Here's how the part is built. I have some questions about the finished solid (model axes, mm). A direction names the side the tool comes from. Give positions to 0.01 mm unless a question says otherwise; leave off trailing zeros. Loops run counter-clockwise (first coordinate to the right, second up) from the corner with the lowest first, then second, coordinate; pieces in that order, holes last. Notation, with made-up numbers: (61.5, -16) - (82.5, -16) arc R17 ccw to (82.5, 16) - close; hole circle Ø11 at (-20, 58). An arc over 180 degrees is marked (long way). Return JSON: item names as keys, results as strings. Group by question number.
(1) I need wall thicknesses on probe 1 along X at (y, z) = (12.75, -0.1); probe 2 along Y at (x, z) = (-1.5, 0.95); probe 3 along Z at (x, y) = (-0.5, 22). Which ranges of each line are inside material? Lowest first, please. Write a range as [from, to].
(2) If we section it at C-C (z = 1.25): Please give me the cut outline in (x, y), then the cut area to 3 significant figures.
(3) If we mould it in two halves opening along Y, with no side actions, what happens to faces 1 (the cylindrical face through (1, 10, 0)), 2 (the flat face through (1, 22.209, 1)), 3 (the flat face through (1, 20, 1))? For each: released by +Y, released by -Y, zero draft, split by the parting line, or undercut.
(4) On a 3-axis mill with a long thin cutter (end or side, diameter ignored), from which of +Z, -Z, +X, -X, +Y, -Y can I reach the whole of each face in a straight line? I mean faces 4 (the cylindrical face through (1, 22, 0)), 5 (the cylindrical face through (2, 21, 0)). Say none if no direction works.
(5) For P1, Ø2, axis at y = 4.5, z = -1.5, coming from the +X side; P2, Ø2, axis at y = 17.5, z = 0, coming from the +X side, each with a flat end and sliding along its axis, tell me the tip position at first contact or that it passes through.
(6) If we section it at A-A (x = 0): Please give me the cut outline in (y, z), then the cut area to 3 significant figures.
(7) If we section it at D-D (y = 9.75): Please give me the cut outline in (x, z).
(8) If we section it at B-B (z = 0): Please give me the cut outline in (x, y), then the cut area to 3 significant figures.
```python
from build123d import *


with BuildPart() as part:
    # Sketch1 → Screw Revolve (revolve)
    with BuildSketch(Plane.XY, mode=Mode.PRIVATE) as screw_revolve_sk:
        with BuildLine():
            Line((0, 0), (1, 0))
            Line((1, 0), (1, 20))
            Line((1, 20), (2, 20))
            Line((2, 20), (2, 21.209302326))
            Line((2, 21.209302326), (1, 21.209302326))
            Line((1, 21.209302326), (1, 22.209302326))
            Line((1, 22.209302326), (2, 22.209302326))
            ThreePointArc((2, 22.209302326), (1.414213562, 23.623515888), (0, 24.209302326))
            Line((0, 24.209302326), (0, 0))
        make_face()
    revolve(screw_revolve_sk.sketch.rotate(Axis((0, 0, 0), (0, 1, 0)), 90), axis=Axis((0, 0, 0), (0, 1, 0)))


solid = part.part
```
Values:
{
 "1": {"probe 1": "[-0.99, 0.99]", "probe 2": "[20, 21.21], [22.21, 23.13]", "probe 3": "[-0.87, 0.87]"},
 "2": {"outline": "(-1.56, 20) - (1.56, 20) - (1.56, 21.21) - (-1.56, 21.21) - close; (-1.56, 22.21) - (1.56, 22.21) arc R1.56 ccw to start", "area": "7.60 mm2"},
 "3": {"face 1": "zero draft", "face 2": "undercut", "face 3": "released by -Y"},
 "4": {"face 4": "none", "face 5": "+Y, -Y"},
 "5": {"P1": "x = 0.87", "P2": "x = 1"},
 "6": {"outline": "(0, -1) - (20, -1) - (20, -2) - (21.21, -2) - (21.21, -1) - (22.21, -1) - (22.21, -2) arc R2 ccw to (22.21, 2) - (22.21, 1) - (21.21, 1) - (21.21, 2) - (20, 2) - (20, 1) - (0, 1) - close", "area": "53.1 mm2"},
 "7": {"outline": "circle Ø2 at (0, 0)"},
 "8": {"outline": "(-2, 20) - (-1, 20) - (-1, 0) - (1, 0) - (1, 20) - (2, 20) - (2, 21.21) - (1, 21.21) - (1, 22.21) - (2, 22.21) arc R2 ccw to (-2, 22.21) - (-1, 22.21) - (-1, 21.21) - (-2, 21.21) - close", "area": "53.1 mm2"}
}
